CAD build for the part. Positions are in the model's coordinates, mm. A direction names the side the tool comes from. Round coordinates to 2 decimals unless told otherwise and drop trailing zeros. Write each loop counter-clockwise with the first axis right and the second up, starting at its lowest first coordinate (ties: lowest second). Pieces come first, ordered by that corner, then holes. Notation, with made-up numbers: (-4.5, 49) - (16.5, 49) arc R21 cw to (16.5, 59) - close; hole circle Ø1 at (57.25, -7.75). An arc over 180 degrees is marked (long way). Answer in a Markdown table with one row per item.
```python
from build123d import *

# Parameters (mm, degrees)
F2_R     = 4.7879
F3_DEPTH = 9.5758
F4_R     = 5.08
F5_R     = 1.5875
F6_DEPTH = 21.6662


with BuildPart() as f1:
    # F0 (on Front) → F1 (revolve)
    with BuildSketch(Plane.XZ):
        Polygon((0, 48.886847), (0, 0), (31.123154, 7.487174), (31.123154, 48.886847), (11.450971, 38.610332), (11.450971, 48.886847), align=None)
    revolve(axis=Axis((0, 0, 24.443423), (0, 0, 1)))

    # F2 (on face) → F3 (cut)
    with BuildSketch(Plane.XY.offset(48.886847)):
        Circle(F2_R)
    extrude(amount=-F3_DEPTH, mode=Mode.SUBTRACT)

    # F4
    f4_edges = [f1.edges().sort_by_distance(p)[0] for p in [
        (-31.123154, 0, 7.487174),
        (-31.123154, 0, 48.886847),
        (31.123154, 0, 28.18701),
        (-11.450971, 0, 48.886847),
    ]]
    fillet(f4_edges, radius=F4_R)

    # F5 (on Top) → F6 (cut)
    with BuildSketch(Plane.XY):
        Circle(F5_R)
    extrude(amount=F6_DEPTH, mode=Mode.SUBTRACT)


solid = f1.part
```
Q1. Pull direction Y, two halves, no side cores. Call faces 3 (the cylindrical face through (-1.491, 11.354, 41.245)), 4 (the cylindrical face through (-31.093, 1.368, 26.199)), 5 (the flat face through (1, 5, 48.887)): released by +Y, released by -Y, zero draft, split by the parting line, or undercut.
Computed:
| item | result |
|---|---|
| face 3 | undercut |
| face 4 | split by the parting line |
| face 5 | zero draft |
Q2. 3-axis set-ups, long thin cutter, end or side, ignore diameter. For faces 1 (the flat face through (0, 0, 21.666)), 2 (the flat face through (0, 0, 39.311)): which of +Z, -Z, +X, -X, +Y, -Y reach the whole face in a straight line?
Computed:
| item | result |
|---|---|
| face 1 | -Z |
| face 2 | +Z |
Q3. Saw through at A-A on z = 35. List the corners of the cut face in (x, y), then the cut area to 3 significant figures.
Computed:
| item | result |
|---|---|
| outline | circle Ø62.25 at (0, 0) |
| area | 3,040 mm2 |
Q4. Drill centre lines: line 1 (X direction, y = -4, z = 41); line 2 (Y direction, x = 0, z = 45); line 3 (Y direction, x = 0, z = 44.75). Where is each one in solid material? Low to high.
Computed:
| item | result |
|---|---|
| line 1 | x = -30.84 to -15.52, -10.73 to -2.63, 2.63 to 10.73, 15.52 to 30.84 |
| line 2 | y = -28.4 to -23.68, -11.31 to -4.79, 4.79 to 11.31, 23.68 to 28.4 |
| line 3 | y = -28.83 to -23.2, -11.36 to -4.79, 4.79 to 11.36, 23.2 to 28.83 |
Q5. Flat gauge pins, fed straight in: pin 1 (6 mm diameter, centred on x = -9, y = 17.5, fed in from +Z); pin 2 (1 mm diameter, centred on x = -1, z = 9.5, fed in from -Y); pin 3 (12 mm diameter, centred on x = 7.5, z = 35.5, fed in from +Y). Where does each tip first touch, or does it go through?
Computed:
| item | result |
|---|---|
| pin 1 | stops at z = 44.48 |
| pin 2 | stops at y = -30.88 |
| pin 3 | stops at y = 31.09 |
